Could you check a few things on this model? Use its own coordinates, in mm. A direction names the side the tool comes from. Coordinates: 2 decimals unless noted, no trailing zeros. Write each loop counter-clockwise with the first axis right and the second up, starting at its lowest first coordinate (ties: lowest second). Pieces come first, ordered by that corner, then holes. Notation, with made-up numbers: (80, 22.25) - (117, 22.25) arc R17 cw to (117, 30.25) - close; hole circle Ø9 at (-38.5, -13). An arc over 180 degrees is marked (long way). Answer as a JSON object with one key per item and string values. Group by question number.
1) If we section it at C-C (x = 8.25): Write out the boundary of the cut face in (y, z).
2) We'd pull the mould along X, two halves only. Please class faces 1 (the flat face through (2, 1, 1)), 2 (the flat face through (-9, -12, 2)), 3 (the flat face through (5, -9.5, 2)): released by +X, released by -X, zero draft, split by the parting line, or undercut.
3) If we section it at D-D (y = -14): Write out the boundary of the cut face in (x, z).
4) If we section it at A-A (z = 2.5): Write out the boundary of the cut face in (x, y).
5) Will these pins go through, and if not, where does the flat tip stop? pin 1 Ø3 at (x, z) = (-6.5, 2.5) entering from +Y; pin 2 Ø2 at (y, z) = (-4, 1.5) entering from +X; pin 3 Ø0.8 at (y, z) = (2, 0.5) entering from -X.
6) If we section it at B-B (y = -9.25): Write out the boundary of the cut face in (x, z), plus the area to 3 significant figures.
7) On a 3-axis mill with a long thin cutter (end or side, diameter ignored), from which of +Z, -Z, +X, -X, +Y, -Y can I reach the whole of each face in a straight line? I mean faces 4 (the flat face through (0, 1, 1.5)), 5 (the flat face through (2, -8, 2)), 6 (the flat face through (4.5, -5, 2)), 7 (the flat face through (-4.5, -4, 2)). Say none if no direction works.
8) Please list where these lines run through material, in increasing order: line 1 along Z through (x, y) = (7.9, -14); line 2 along X through (y, z) = (-6.25, 0.6); line 3 along X through (y, z) = (-12, 2.8).
```python
from build123d import *

# Parameters (mm, degrees)
F0_W     = 4
F0_H     = 7.5
F1_DEPTH = 1.5
F2_DEPTH = 5
F4_D     = 3
F5_R     = 1


with BuildPart() as f1:
    # F0 (on Top) → F1 (new body)
    with BuildSketch(Plane.XY):
        with Locations((0, 1.25)):
            Rectangle(F0_W, F0_H)
        Polygon((4.5, -2.5), (2, -2.5), (-2, -2.5), (-4.5, -2.5), (-4.5, -7.5), (-9, -7.5), (-9, -9.5), (-9, -16.5), (-7.5, -16.5), (-7.5, -9.5), (-2, -9.5), (-2, -5), (2, -5), (2, -9.5), (7.5, -9.5), (7.5, -16.5), (9, -16.5), (9, -9.5), (9, -7.5), (4.5, -7.5), align=None)
    extrude(amount=F1_DEPTH)

    # F0 (on Top) → F2 (join)
    with BuildSketch(Plane.XY):
        Polygon((4.5, -2.5), (2, -2.5), (-2, -2.5), (-4.5, -2.5), (-4.5, -7.5), (-9, -7.5), (-9, -9.5), (-9, -16.5), (-7.5, -16.5), (-7.5, -9.5), (-2, -9.5), (-2, -5), (2, -5), (2, -9.5), (7.5, -9.5), (7.5, -16.5), (9, -16.5), (9, -9.5), (9, -7.5), (4.5, -7.5), align=None)
    extrude(amount=F2_DEPTH)

    # F4 (through all)
    with Locations(Plane(origin=(-9, 0, 0), x_dir=(0, -1, 0), z_dir=(-1, 0, 0))):
        with Locations((14, 2.5)):
            Hole(F4_D / 2)

    # F5
    f5_edges = [f1.edges().sort_by_distance(p)[0] for p in [
        (2, -5, 2.5),
        (-2, -5, 2.5),
        (-4.5, -7.5, 2.5),
        (4.5, -7.5, 2.5),
    ]]
    fillet(f5_edges, radius=F5_R)


solid = f1.part
```
Here are the results:
{
 "1": {"outline": "(-16.5, 0) - (-7.5, 0) - (-7.5, 5) - (-16.5, 5) - close; hole circle Ø3 at (-14, 2.5)"},
 "2": {"face 1": "released by +X", "face 2": "released by -X", "face 3": "undercut"},
 "3": {"outline": "(-9, 0) - (-7.5, 0) - (-7.5, 1) - (-9, 1) - close; (-9, 4) - (-7.5, 4) - (-7.5, 5) - (-9, 5) - close; (7.5, 0) - (9, 0) - (9, 1) - (7.5, 1) - close; (7.5, 4) - (9, 4) - (9, 5) - (7.5, 5) - close"},
 "4": {"outline": "(-9, -16.5) - (-7.5, -16.5) - (-7.5, -15.5) - (-9, -15.5) - close; (-9, -12.5) - (-7.5, -12.5) - (-7.5, -9.5) - (-2, -9.5) - (-2, -6) arc R1 cw to (-1, -5) - (1, -5) arc R1 cw to (2, -6) - (2, -9.5) - (7.5, -9.5) - (7.5, -12.5) - (9, -12.5) - (9, -7.5) - (5.5, -7.5) arc R1 cw to (4.5, -6.5) - (4.5, -2.5) - (-4.5, -2.5) - (-4.5, -6.5) arc R1 cw to (-5.5, -7.5) - (-9, -7.5) - close; (7.5, -16.5) - (9, -16.5) - (9, -15.5) - (7.5, -15.5) - close"},
 "5": {"pin 1": "stops at y = -7.37", "pin 2": "stops at x = 4.5", "pin 3": "stops at x = -2"},
 "6": {"outline": "(-9, 0) - (-2, 0) - (-2, 5) - (-9, 5) - close; (2, 0) - (9, 0) - (9, 5) - (2, 5) - close", "area": "70.0 mm²"},
 "7": {"face 4": "+Z, +X, -X, +Y", "face 5": "+Z, -Z, -Y", "face 6": "+Z, -Z, +X, +Y", "face 7": "+Z, -Z, -X, +Y"},
 "8": {"line 1": "z = 0 to 1, 4 to 5", "line 2": "x = -4.5 to -2, 2 to 4.5", "line 3": "x = -9 to -7.5, 7.5 to 9"}
}
